from build123d import *

# Parameters (mm, degrees)
F0_W      = 97.79
F0_H      = 97.79
F1_DEPTH  = 1.5875
F2_W      = 97.79
F2_H      = 96.2025
F2_H_2    = 1.5875
F3_DEPTH  = 1.5875
F4_W      = 97.79
F4_H      = 99.3775
F5_DEPTH  = 1.5875
F6_W      = 96.2025
F6_H      = 99.3775
F6_W_2    = 1.5875
F7_DEPTH  = 1.5875
F8_R      = 4
F9_DEPTH  = 25.4
F10_W     = 96.2025
F10_H     = 97.79
F10_W_2   = 1.5875
F11_DEPTH = 1.5875
F12_W     = 97.79
F12_H     = 97.79
F13_DEPTH = 1.5875


with BuildPart() as f1:
    # F0 (on Front) → F1 (new body)
    with BuildSketch(Plane.XZ):
        Rectangle(F0_W, F0_H)
    extrude(amount=F1_DEPTH)

    # F2 (on face) → F3 (join)
    with BuildSketch(Plane.XY.offset(48.895)):
        with Locations((0, -49.68875)):
            Rectangle(F2_W, F2_H)
        with Locations((0, -0.79375)):
            Rectangle(F2_W, F2_H_2)
    extrude(amount=F3_DEPTH)

    # F4 (on face) → F5 (join)
    with BuildSketch(Plane(origin=(0, 0, 0), x_dir=(-1, 0, 0), z_dir=(0, 1, 0))):
        with Locations((0, 0.79375)):
            Rectangle(F4_W, F4_H)
    extrude(amount=F5_DEPTH)

    # F6 (on face) → F7 (join)
    with BuildSketch(Plane.YZ.offset(48.895)):
        with Locations((49.68875, 0.79375)):
            Rectangle(F6_W, F6_H)
        with Locations((0.79375, 0.79375)):
            Rectangle(F6_W_2, F6_H)
    extrude(amount=F7_DEPTH)

    # F8 (on face) → F9 (cut)
    with BuildSketch(Plane.YZ.offset(50.4825)):
        with Locations((48.895, 0)):
            Circle(F8_R)
    extrude(amount=-F9_DEPTH, mode=Mode.SUBTRACT)

    # F10 (on face) → F11 (join)
    with BuildSketch(Plane.XZ):
        with Locations((98.58375, 0)):
            Rectangle(F10_W, F10_H)
        with Locations((49.68875, 0)):
            Rectangle(F10_W_2, F10_H)
    extrude(amount=F11_DEPTH)

    # F12 (on face) → F13 (join)
    with BuildSketch(Plane.YZ.offset(50.4825)):
        with Locations((-48.895, 0)):
            Rectangle(F12_W, F12_H)
    extrude(amount=F13_DEPTH)


solid = f1.part
Here's how the part is built. I have some questions about the finished solid (model axes, mm). A direction names the side the tool comes from. Coordinates: 2 decimals unless noted, no trailing zeros. Write each loop counter-clockwise with the first axis right and the second up, starting at its lowest first coordinate (ties: lowest second). Pieces come first, ordered by that corner, then holes.
1) If we section it at B-B (z = 0): List the corners of the cut face in (x, y) for me (1 decimal), plus the area to 3 significant figures.
Filled in:
outline: (-48.9, -1.6) - (50.5, -1.6) - (50.5, -97.8) - (52.1, -97.8) - (52.1, -1.6) - (146.7, -1.6) - (146.7, 0) - (50.5, 0) - (50.5, 44.9) - (48.9, 44.9) - (48.9, 1.6) - (-48.9, 1.6) - close; (48.9, 52.9) - (50.5, 52.9) - (50.5, 97.8) - (48.9, 97.8) - close
area: 761 mm2
2) If we section it at A-A (y = -59.5): List the corners of the cut face in (x, z) for me (1 decimal), plus the area to 3 significant figures.
Filled in:
outline: (-48.9, 48.9) - (48.9, 48.9) - (48.9, 50.5) - (-48.9, 50.5) - close; (50.5, -48.9) - (52.1, -48.9) - (52.1, 48.9) - (50.5, 48.9) - close
area: 310 mm2
3) Which directions (+Z, -Z, +X, -X, +Y, -Y) give clear straight access to the entire face, cutting with the end or side of a thin tool? Please do faces 4 (the face through (50.482, -50, 1)), 5 (the face through (98, 0, 1)), 6 (the face through (1, 1.588, 1)), 7 (the face through (-1, -49, 48.895)).
Filled in:
face 4: +Z, -Z, -X, -Y
face 5: +Z, -Z, +X, +Y
face 6: +Z, -Z, -X, +Y
face 7: -Z, -X, -Y
4) I'm going to push flat-ended pins straight in: pin 1 (5 mm diameter, centred on y = 48.895, z = 0, fed in from -X); pin 2 (8 mm diameter, centred on x = 20, z = -13, fed in from -Y); pin 3 (0.8 mm diameter, centred on x = 49.5, z = 49.5, fed in from -Y); pin 4 (1 mm diameter, centred on y = 16.5, z = 19, fed in from +X). Where does each tip first touch, or does it pass through?
Filled in:
pin 1: passes through
pin 2: stops at y = -1.59
pin 3: stops at y = 0
pin 4: stops at x = 50.48
5) If I drill on line 1 (Y direction, x = 109.5, z = 6.5); line 2 (X direction, y = 12, z = 7.5) (1 decimal), over which ranges is the centre line in solid material (lowest first)?
Filled in:
line 1: y = -1.59 to 0
line 2: x = 48.9 to 50.5
6) If we section it at D-D (z = -16): List the corners of the cut face in (x, y) for me (1 decimal), plus the area to 3 significant figures.
Filled in:
outline: (-48.9, -1.6) - (50.5, -1.6) - (50.5, -97.8) - (52.1, -97.8) - (52.1, -1.6) - (146.7, -1.6) - (146.7, 0) - (50.5, 0) - (50.5, 97.8) - (48.9, 97.8) - (48.9, 1.6) - (-48.9, 1.6) - close
area: 774 mm2
7) If we section it at C-C (x = -10.5): List the corners of the cut face in (y, z) for me (1 decimal), plus the area to 3 significant figures.
Filled in:
outline: (-97.8, 48.9) - (-1.6, 48.9) - (-1.6, -48.9) - (1.6, -48.9) - (1.6, 50.5) - (-97.8, 50.5) - close
area: 468 mm2
8) Thinking about a two-plate mould opening in Y: for faces 1 (the face through (49.7, 44.9, 0.2)), 2 (the face through (52.07, -50, 1)), 3 (the face through (0, -1.588, 1)), which applies, +Y half, -Y half, draft (parallel to the pull), parting line (faces both ways), or undercut?
Filled in:
face 1: undercut
face 2: draft
face 3: -Y half
